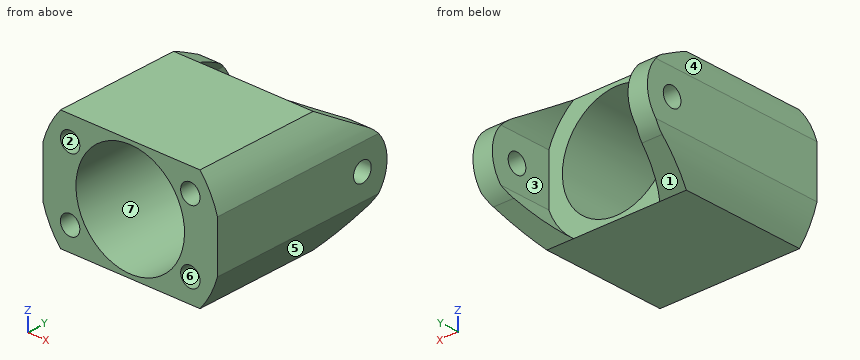
```python
from build123d import *

# Parameters (mm, degrees)
SKETCH1_R              = 14
BOSS_EXTRUDE1_DEPTH    = 32
BOSS_EXTRUDE2_DEPTH    = 45
SKETCH4_R              = 49.397099685
SKETCH4_R_2            = 14
CUT_EXTRUDE1_DEPTH     = 90
FILLET1_R              = 10
SKETCH6_R              = 2.5
CUT_EXTRUDE2_DEPTH     = 90
CUT_EXTRUDE3_START     = -18
CUT_EXTRUDE3_OUTLINE_R = 14
CUT_EXTRUDE3_DEPTH     = 17
SKETCH8_R              = 2.5
CUT_EXTRUDE4_DEPTH     = 6


with BuildPart() as part:
    # Sketch1 → Boss-Extrude1 (new body)
    with BuildSketch(Plane(origin=(0, 0, 0), x_dir=(1, 0, 0), z_dir=(0, 1, 0))):
        with BuildLine():
            ThreePointArc((-22.5, -6.5), (-20.684382748, -10.984366633), (-17.986105749, -15))
            Line((-17.986105749, -15), (17.986105749, -15))
            ThreePointArc((17.986105749, -15), (20.684382748, -10.984366633), (22.5, -6.5))
            Line((22.5, -6.5), (22.5, 6.5))
            ThreePointArc((22.5, 6.5), (20.684382748, 10.984366633), (17.986105749, 15))
            Line((17.986105749, 15), (-17.986105749, 15))
            ThreePointArc((-17.986105749, 15), (-20.684382748, 10.984366633), (-22.5, 6.5))
            Line((-22.5, 6.5), (-22.5, -6.5))
        make_face()
        with Locations(Location((0, 0, 0), (0, 0, 270))):
            Circle(SKETCH1_R, mode=Mode.SUBTRACT)
    extrude(amount=BOSS_EXTRUDE1_DEPTH)

    # Sketch3 → Boss-Extrude2 (add)
    with BuildSketch(Plane(origin=(22.5, 0, 0), x_dir=(0, 0, -1), z_dir=(1, 0, 0))):
        Polygon((-15, 32), (15, 32), (0, 57.980762114), align=None)
    extrude(amount=-BOSS_EXTRUDE2_DEPTH)

    # Sketch4 → Cut-Extrude1 (cut)
    # profile 1 of 2: a face of its own
    with BuildSketch(Plane.XZ):
        Circle(SKETCH4_R)
        with BuildLine():
            ThreePointArc((22.5, 6.5), (23.188916849, 3.282397806), (23.420076857, 0))
            ThreePointArc((23.420076857, 0), (23.188916849, -3.282397806), (22.5, -6.5))
            ThreePointArc((22.5, -6.5), (20.684382748, -10.984366633), (17.986105749, -15))
            ThreePointArc((17.986105749, -15), (0, -23.420076857), (-17.986105749, -15))
            ThreePointArc((-17.986105749, -15), (-20.684382748, -10.984366633), (-22.5, -6.5))
            ThreePointArc((-22.5, -6.5), (-23.420076857, 0), (-22.5, 6.5))
            ThreePointArc((-22.5, 6.5), (-20.684382748, 10.984366633), (-17.986105749, 15))
            ThreePointArc((-17.986105749, 15), (0, 23.420076857), (17.986105749, 15))
            ThreePointArc((17.986105749, 15), (20.684382748, 10.984366633), (22.5, 6.5))
        make_face(mode=Mode.SUBTRACT)
    # profile 2 of 2: a face of its own
    with BuildSketch(Plane.XZ):
        Circle(SKETCH4_R_2)
    extrude(amount=-CUT_EXTRUDE1_DEPTH, mode=Mode.SUBTRACT)

    # Fillet1
    # the kernel refuses this fillet: 10 mm, written as the material it takes off along each edge
    with BuildSketch(Plane(origin=(29.301270189, 57.980762114, 0), x_dir=(0, -0.8660254037844386, -0.5), z_dir=(-1, 0, 0)), Plane(origin=(65.801270189, 57.980762114, 0), x_dir=(0, -0.8660254037844386, -0.5), z_dir=(-1, 0, 0))) as fillet1_piece_1:
        with BuildLine():
            CenterArc((FILLET1_R * 1.73205080757, FILLET1_R), FILLET1_R, 150, 120)
            Line((FILLET1_R * 0.866025403784, FILLET1_R * 1.5), (0, 0))
            Line((0, 0), (FILLET1_R * 1.73205080757, 0))
        make_face()
    extrude(amount=95.102540378, mode=Mode.SUBTRACT)

    # Sketch6 → Cut-Extrude2 (cut)
    with BuildSketch(Plane.ZY.offset(22.5)):
        with Locations((0, 41)):
            Circle(SKETCH6_R)
    extrude(amount=-CUT_EXTRUDE2_DEPTH, mode=Mode.SUBTRACT)

    # Cut-Extrude3: read off the stored shape, not the designer's step
    # Cut-Extrude3 outline → Cut-Extrude3 (cut)
    with BuildSketch(Plane(origin=(0, 50, 0), x_dir=(1, 0, 0), z_dir=(0, 1, 0)).offset(CUT_EXTRUDE3_START)):
        with BuildLine():
            ThreePointArc((-17.5, -6.5), (-14.924450898, -11.21431074), (-11.113055385, -15))
            Line((-11.113055385, -15), (11.113055385, -15))
            ThreePointArc((11.113055385, -15), (14.924450898, -11.21431074), (17.5, -6.5))
            Line((17.5, -6.5), (17.5, 6.5))
            ThreePointArc((17.5, 6.5), (14.924450898, 11.21431074), (11.113055385, 15))
            Line((11.113055385, 15), (-11.113055385, 15))
            ThreePointArc((-11.113055385, 15), (-14.924450898, 11.21431074), (-17.5, 6.5))
            Line((-17.5, 6.5), (-17.5, -6.5))
        make_face()
        Circle(CUT_EXTRUDE3_OUTLINE_R, mode=Mode.SUBTRACT)
    extrude(amount=CUT_EXTRUDE3_DEPTH, mode=Mode.SUBTRACT)

    # Sketch8 → Cut-Extrude4 (cut)
    with BuildSketch(Plane.XZ):
        with Locations(Location((-15.5, 9, 0), (0, 0, 270))):
            Circle(SKETCH8_R)
        with Locations(Location((15.5, 9, 0), (0, 0, 270))):
            Circle(SKETCH8_R)
        with Locations(Location((15.5, -9, 0), (0, 0, 270))):
            Circle(SKETCH8_R)
        with Locations(Location((-15.5, -9, 0), (0, 0, 270))):
            Circle(SKETCH8_R)
    extrude(amount=-CUT_EXTRUDE4_DEPTH, mode=Mode.SUBTRACT)


solid = part.part
```
Model file for the job. Use its own axes, mm. Face numbers are marked on the shaded views. A direction names the side the tool comes from. Coordinates: 2 decimals unless noted, no trailing zeros. Write each loop counter-clockwise with the first axis right and the second up, starting at its lowest first coordinate (ties: lowest second). Pieces come first, ordered by that corner, then holes. Notation, with made-up numbers: (10, 33.25) - (68, 33.25) arc R15 ccw to (68, 51.25) - close; hole circle Ø1 at (67.5, 68). An arc over 180 degrees is marked (long way). One line per item, written item: value. Start each with the question number.
1. Slice it at A-A (y = 25). Write the cut outline in (x, z).
2. Tool access for the marked faces 1, 2 and 3: list every direction of +Z, -Z, +X, -X, +Y, -Y with a clear straight run to the whole face (end or side of a thin tool).
3. Flat gauge pins, fed straight in: pin 1 (2.5 mm diameter, centred on x = 15.5, z = -8, fed in from -Y); pin 2 (2 mm diameter, centred on y = 38.5, z = -10, fed in from +X); pin 3 (6 mm diameter, centred on x = -15.5, z = 9, fed in from -Y); pin 4 (1.5 mm diameter, centred on y = 31.5, z = 11, fed in from +X). Where does each tip first touch, or does it go through?
4. Slice it at B-B (z = 0). Write the cut outline in (x, y).
5. Probe line 1 (X direction, y = 37, z = -5.5); line 2 (X direction, y = 30.5, z = -0.5); line 3 (Z direction, x = 15, y = 4). List the from-to ranges inside material, lowest first. Write a range as from..to.
6. Slice it at C-C (x = -10). Write the cut outline in (y, z).
7. Mould opens along Z. For the marked faces 4, 5, 6 and 7 say: released by +Z, released by -Z, zero draft, split by the parting line, or undercut.
8. Slice it at D-D (y = 41). Write the cut outline in (x, z), plus the area to 3 significant figures.
Answers below:
1. outline: (-22.5, -6.5) arc R23.42 ccw to (-17.99, -15) - (17.99, -15) arc R23.42 ccw to (22.5, -6.5) - (22.5, 6.5) arc R23.42 ccw to (17.99, 15) - (-17.99, 15) arc R23.42 ccw to (-22.5, 6.5) - close; hole circle Ø28 at (0, 0)
2. face 1: -Z, +X, -X, +Y
2. face 2: -Y
2. face 3: +Y
3. pin 1: stops at y = 6
3. pin 2: stops at x = 21.62
3. pin 3: stops at y = 0
3. pin 4: stops at x = 21.06
4. outline: (-22.5, 0) - (-14, 0) - (-14, 32) - (-17.5, 32) - (-17.5, 38.5) - (-22.5, 38.5) - close; (-22.5, 43.5) - (-17.5, 43.5) - (-17.5, 47.98) - (-22.5, 47.98) - close; (14, 0) - (22.5, 0) - (22.5, 38.5) - (17.5, 38.5) - (17.5, 32) - (14, 32) - close; (17.5, 43.5) - (22.5, 43.5) - (22.5, 47.98) - (17.5, 47.98) - close
5. line 1: x = -22.5..-17.5, 17.5..22.5
5. line 2: x = -22.5..-13.99, 13.99..22.5
5. line 3: z = -15..-11.45, -6.55..6.55, 11.45..15
6. outline: (0, -15) - (32, -15) - (32, -9.8) - (0, -9.8) - close; (0, 9.8) - (32, 9.8) - (32, 15) - (0, 15) - close
7. face 4: released by +Z
7. face 5: released by -Z
7. face 6: undercut
7. face 7: undercut
8. outline: (-22.5, -6.5) arc R23.42 ccw to (-21.27, -9.8) - (-15.89, -9.8) arc R18.67 cw to (-17.5, -6.5) - (-17.5, -2.5) - (-22.5, -2.5) - close; (-22.5, 2.5) - (-17.5, 2.5) - (-17.5, 6.5) arc R18.67 cw to (-15.89, 9.8) - (-21.27, 9.8) arc R23.42 ccw to (-22.5, 6.5) - close; (15.89, -9.8) - (21.27, -9.8) arc R23.42 ccw to (22.5, -6.5) - (22.5, -2.5) - (17.5, -2.5) - (17.5, -6.5) arc R18.67 cw to start; (15.89, 9.8) arc R18.67 cw to (17.5, 6.5) - (17.5, 2.5) - (22.5, 2.5) - (22.5, 6.5) arc R23.42 ccw to (21.27, 9.8) - close
8. area: 148 mm^2
